Autodesk Inventor part; units mm, degrees
ref_plane "YZ Plane" through (0, 0, 0) normal (1, 0, 0) x (0, 1, 0)
ref_plane "XZ Plane" through (0, 0, 0) normal (0, 1, 0) x (-1, 0, 0)
ref_plane "XY Plane" through (0, 0, 0) normal (0, 0, 1) x (1, 0, 0)
sketch "Sketch1" plane through (0, 0, 0) normal (0, 1, 0) x (-1, 0, 0)
  line L0 (-1.4605, -5.842) -> (-2.0955, -5.842)
  line L1 (-2.0955, -5.842) -> (-2.0955, 4.3815)
  line L2 (-2.0955, 4.3815) -> (2.286, 4.3815)
  line L3 (2.286, 4.3815) -> (2.286, 3.7465)
  line L4 (2.286, 3.7465) -> (-1.4605, 3.7465)
  line L5 (-1.4605, 3.7465) -> (-1.4605, -5.842)
  line L6 (2.286, 6.2865) -> (2.286, 6.9215)
  line L7 (2.286, 6.9215) -> (-4.6355, 6.9215)
  line L8 (-4.6355, 6.9215) -> (-4.6355, -5.842)
  line L9 (-4.6355, -5.842) -> (-4.0005, -5.842)
  line L10 (-4.0005, -5.842) -> (-4.0005, 6.2865)
  line L11 (-4.0005, 6.2865) -> (2.286, 6.2865)
  line L12 (2.286, 8.8265) -> (2.286, 9.4615)
  line L13 (2.286, 9.4615) -> (-7.1755, 9.4615)
  line L14 (-7.1755, 9.4615) -> (-7.1755, -5.842)
  line L15 (-7.1755, -5.842) -> (-6.5405, -5.842)
  line L16 (-6.5405, -5.842) -> (-6.5405, 8.8265)
  line L17 (-6.5405, 8.8265) -> (2.286, 8.8265)
  line L18 (2.286, 4.064) -> (9.1077, 4.064) construction
  line L19 (2.286, 6.604) -> (8.649, 6.604) construction
  line L20 (2.286, 9.144) -> (8.4197, 9.144) construction
  line L21 (-1.778, -5.842) -> (-1.778, -10.327) construction
  line L22 (-4.318, -5.842) -> (-4.318, -10.188) construction
  line L23 (-6.858, -5.842) -> (-6.858, -10.8865) construction
  line L24 (12.5548, 0) -> (-11.5751, 0) construction
  line L25 (0, -14.9561) -> (0, 13.5311) construction
  line L26 (0, 0) -> (-8.128, 0) construction
  line L27 (-8.128, 0) -> (-8.128, 2.54) construction
  line L28 (-8.128, 2.54) -> (0, 2.54) construction
  line L29 (0, 2.54) -> (0, 0) construction
  line L30 (-2.54, 0) -> (-2.54, 2.54) construction
  dimension "d24" = 2.54
  dimension "d25" = 2.54
  dimension "d26" = 2.54
  dimension "d27" = 2.54
  dimension "d29" = 0.635
  dimension "d30" = 5.842
  dimension "d32" = 2.54
  dimension "d33" = 8.128
  dimension "d34" = 2.286
  dimension "d35" = 1.778
  dimension "d36" = 1.524
  dimension "d44" = 2.54
  dimension "d45" = 4.826
extrude "Extrusion1" add sketch "Sketch1" along normal mid plane 0.635
sketch "Sketch3" plane through (0, 0, 0) normal (0, 0, 1) x (1, 0, 0)
  line L0 (0, -1.27) -> (8.128, -1.27)
  line L1 (8.128, -1.27) -> (8.128, 1.27)
  line L2 (8.128, 1.27) -> (0, 1.27)
  line L3 (0, 1.27) -> (0, -1.27)
  line L4 (1.4605, 0.3175) -> (1.4605, -0.3175)
  line L5 (1.4605, -0.3175) -> (1.4605, 0.3175)
  line L6 (2.0955, 0.3175) -> (1.4605, 0.3175)
  line L7 (1.4605, 0.3175) -> (-2.286, 0.3175)
  line L8 (-2.286, 0.3175) -> (2.0955, 0.3175)
  line L9 (1.4605, -0.3175) -> (2.0955, -0.3175)
  line L10 (2.0955, -0.3175) -> (-2.286, -0.3175)
  line L11 (-2.286, -0.3175) -> (1.4605, -0.3175)
  line L12 (1.4605, 0) -> (0, 0) construction
  line L13 (7.1755, -0.3175) -> (7.1755, 0.3175) construction
  line L14 (7.1755, -0.3175) -> (7.1755, 0.3175) construction
  point P0 (0, 0)
  dimension "d37" = 2.54
  dimension "d38" = 8.128
  dimension "d39" = 1.4605
  dimension "d40" = 0.9525
extrude "Extrusion3" add sketch "Sketch3" along normal blind 2.54
properties part number "HeaderRight3"
Can you work these out from the model? Positions are in its coordinate system, mm. A direction names the side the tool comes from. Give positions to 0.01 mm unless a question says otherwise; leave off trailing zeros. Write each loop counter-clockwise with the first axis right and the second up, starting at its lowest first coordinate (ties: lowest second). Pieces come first, ordered by that corner, then holes. Notation, with made-up numbers: (49, 31) -> (79, 31) arc R15 ccw to (79, 41) -> close; hole circle Ø8 at (33, 78.5). An arc over 180 degrees is marked (long way). Write item = value, one per line.
(1) Suppose I cut it at C-C on x = 3.5. Write out the boundary of the cut face in (y, z).
Worked out:
outline = (-1.27, 0) -> (1.27, 0) -> (1.27, 2.54) -> (-1.27, 2.54) -> close; (-0.32, 6.29) -> (0.32, 6.29) -> (0.32, 6.92) -> (-0.32, 6.92) -> close; (-0.32, 8.83) -> (0.32, 8.83) -> (0.32, 9.46) -> (-0.32, 9.46) -> close
(2) For faces 1 (the face through (8.128, 0, 1)), 2 (the face through (4, -1.27, 1)), 3 (the face through (0, 0, 1)), 4 (the face through (0, 0.318, 4)), 5 (the face through (2.5, -0.318, 6.5)), which set-ups out of +Z, -Z, +X, -X, +Y, -Y let a thin tool reach every point of the face, with its end or its side?
Worked out:
face_1 = +Z, -Z, +X, +Y, -Y
face_2 = +Z, -Z, +X, -X, -Y
face_3 = -Z, -X, +Y, -Y
face_4 = +Z, +X, -X, +Y
face_5 = +Z, +X, -X, -Y
(3) Suppose I cut it at B-B on x = 5. Write out the boundary of the cut face in (y, z), then the cut area to 3 significant figures.
Worked out:
outline = (-1.27, 0) -> (1.27, 0) -> (1.27, 2.54) -> (-1.27, 2.54) -> close; (-0.32, 8.83) -> (0.32, 8.83) -> (0.32, 9.46) -> (-0.32, 9.46) -> close
area = 6.85 mm^2
(4) Suppose I cut it at A-A on z = 2.75. Write out the boundary of the cut face in (x, y).
Worked out:
outline = (1.46, -0.32) -> (2.1, -0.32) -> (2.1, 0.32) -> (1.46, 0.32) -> close; (4, -0.32) -> (4.64, -0.32) -> (4.64, 0.32) -> (4, 0.32) -> close; (6.54, -0.32) -> (7.18, -0.32) -> (7.18, 0.32) -> (6.54, 0.32) -> close
(5) I need wall thicknesses on probe 1 along Z at (x, y) = (1.5, 0.25); probe 2 along X at (y, z) = (-0.25, -1.75); probe 3 along Z at (x, y) = (3.5, 0). Which ranges of each line are inside material? Lowest first, please. Write a range as from..to.
Worked out:
probe_1 = -5.84..4.38, 6.29..6.92, 8.83..9.46
probe_2 = 1.46..2.1, 4..4.64, 6.54..7.18
probe_3 = 0..2.54, 6.29..6.92, 8.83..9.46
(6) Thinking about a two-plate mould opening in Z: for faces 6 (the face through (4, -1, 2.54)), 7 (the face through (0, -0.318, 4)), which applies, released by +Z, released by -Z, zero draft, split by the parting line, or undercut?
Worked out:
face_6 = undercut
face_7 = zero draft
(7) I'm going to push flat-ended pins straight in: P1, Ø3, axis at x = 0.5, z = -2, coming from the +Y side; P2, Ø1, axis at x = 0.5, y = -0.5, coming from the -Z side; P3, Ø0.5, axis at y = 0, z = -2, coming from the +X side; P4, Ø0.6, axis at x = 1, z = 3, coming from the +Y side. Where does each tip first touch, or does it pass through?
Worked out:
P1 = 0.32
P2 = 0
P3 = 7.18
P4 = through
